Build history of the part. All positions in model axes, mm. A direction names the side the tool comes from. Give positions to 0.01 mm unless a question says otherwise; leave off trailing zeros. Loops run counter-clockwise (first coordinate to the right, second up) from the corner with the lowest first, then second, coordinate; pieces in that order, holes last. Notation, with made-up numbers: (71.5, -23) -> (75.5, -23) arc R14 cw to (75.5, -3) -> close; hole circle Ø4 at (-7.75, 13.25). An arc over 180 degrees is marked (long way). One line per question, with ' | ' between items. Start each with the question number.
(1) Mould opens along Z. For faces 3 (the face through (-1.29, -12.32, 104.17)), 4 (the face through (-1.29, -87.68, 104.17)), 5 (the face through (0, -75, 59)), 6 (the face through (0.477, -12.325, 116.065)) say: pulls with the +Z half, pulls with the -Z half, needs draft (parallel to the pull), parting line crosses it, or undercut.
(2) Slice it at D-D, the plane x = -12.5. Write the cut outline in (y, z).
(3) Slice it at C-C, the plane y = -89. Write the cut outline in (x, z).
(4) Flat gauge pins, fed straight in: pin 1 Ø22.5 at (x, z) = (0, 94.38) entering from +Y; pin 2 Ø1 at (x, y) = (2.5, -82.5) entering from +Z; pin 3 Ø2 at (y, z) = (-71.5, 15.5) entering from -X. Where does each tip first touch, or does it go through?
(5) Slice it at A-A, the plane z = 36. Write the cut outline in (x, y).
(6) Drill centre lines: L1, parallel to Z at x = 0, y = -91; L2, parallel to X at y = -14.25, z = 0; L3, parallel to Z at x = -2.5, y = -21. Where is each one in solid material? Low to high. Write a range as from..to.
(7) Slice it at B-B, the plane x = 0. Write the cut outline in (y, z).
(8) 3-axis set-ups, long thin cutter, end or side, ignore diameter. For faces 1 (the face through (-21.688, -12, 48)), 2 (the face through (-10.01, -50.7, -19.24)): which of +Z, -Z, +X, -X, +Y, -Y reach the whole face in a straight line?
```python
from build123d import *

# Parameters (mm, degrees)
F0_R     = 9.8737284495
F1_DEPTH = 25
F4_R     = 9.8737284495
F5_DEPTH = 50


with BuildPart() as f1:
    # F0 (on Front) → F1 (new body)
    with BuildSketch(Plane.XZ):
        with BuildLine():
            Line((-21.6877176851, 94.382122159), (-21.6877176851, 0))
            ThreePointArc((-21.6877176851, 0), (0, -21.6877176851), (21.6877176851, 0))
            Line((21.6877176851, 0), (21.6877176851, 94.382122159))
            ThreePointArc((21.6877176851, 94.382122159), (0, 116.0698398441), (-21.6877176851, 94.382122159))
        make_face()
        Circle(F0_R, mode=Mode.SUBTRACT)
        with Locations((0, 94.382122159)):
            Circle(F0_R, mode=Mode.SUBTRACT)
    extrude(amount=F1_DEPTH)


with BuildPart() as f3_1:
    # F3: instance of F1
    add(f1.part.mirror(Plane.XZ.offset(50)))


with BuildPart() as f1_1:
    add(f1.part)

    add(f3_1.part)  # F5 merges F3_1
    # F4 (on face) → F5 (join, through all)
    with BuildSketch(Plane(origin=(0, -75, 0), x_dir=(-1, 0, 0), z_dir=(0, 1, 0))):
        with BuildLine():
            ThreePointArc((-21.6877176851, 0), (0, -21.6877176851), (21.6877176851, 0))
            ThreePointArc((21.6877176851, 0), (0, 21.6877176851), (-21.6877176851, 0))
        make_face()
        Circle(F4_R, mode=Mode.SUBTRACT)
    extrude(amount=F5_DEPTH)


solid = f1_1.part
```
Final values:
1) face 3: undercut | face 4: undercut | face 5: needs draft | face 6: pulls with the +Z half
2) outline: (-100, -17.72) -> (0, -17.72) -> (0, 112.11) -> (-25, 112.11) -> (-25, 17.72) -> (-75, 17.72) -> (-75, 112.11) -> (-100, 112.11) -> close
3) outline: (-21.69, 0) arc R21.69 ccw to (21.69, 0) -> (21.69, 94.38) arc R21.69 ccw to (-21.69, 94.38) -> close; hole circle Ø19.75 at (0, 0); hole circle Ø19.75 at (0, 94.38)
4) pin 1: y = 0 | pin 2: z = 115.98 | pin 3: x = -16.13
5) outline: (-21.69, -100) -> (21.69, -100) -> (21.69, -75) -> (-21.69, -75) -> close; (-21.69, -25) -> (21.69, -25) -> (21.69, 0) -> (-21.69, 0) -> close
6) L1: -21.69..-9.87, 9.87..84.51, 104.26..116.07 | L2: -21.69..-9.87, 9.87..21.69 | L3: -21.54..-9.55, 9.55..84.83, 103.93..115.93
7) outline: (-100, -21.69) -> (0, -21.69) -> (0, -9.87) -> (-100, -9.87) -> close; (-100, 9.87) -> (0, 9.87) -> (0, 84.51) -> (-25, 84.51) -> (-25, 21.69) -> (-75, 21.69) -> (-75, 84.51) -> (-100, 84.51) -> close; (-100, 104.26) -> (-75, 104.26) -> (-75, 116.07) -> (-100, 116.07) -> close; (-25, 104.26) -> (0, 104.26) -> (0, 116.07) -> (-25, 116.07) -> close
8) face 1: +Z, -Z, -X, +Y, -Y | face 2: none
